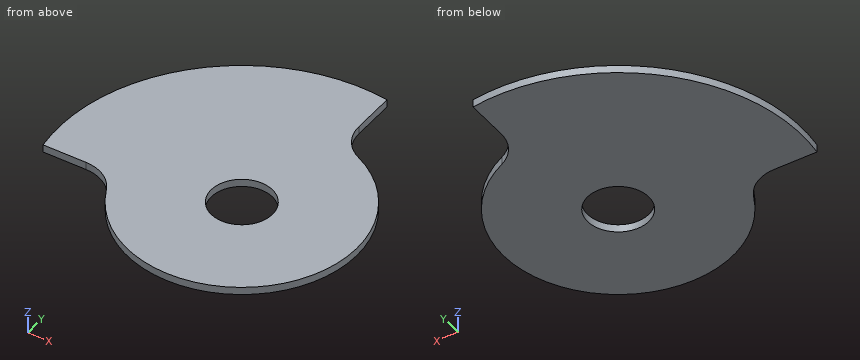
from build123d import *

# Parameters (mm, degrees)
SKETCH_1_R          = 24
EXTRUDE_1_DEPTH     = 1
CUT_EXTRUDE_START   = -1
SKETCH_2_R          = 4
CUT_EXTRUDE_1_DEPTH = 1
FILLET_1_R          = 5
FILLET_2_R          = 5


with BuildPart() as part:
    # 草图1 → 拉伸1 (new body)
    with BuildSketch(Plane.XY):
        Circle(SKETCH_1_R)
    extrude(amount=EXTRUDE_1_DEPTH)

    # 草图2 → 切除-拉伸1 (cut)
    with BuildSketch(Plane.XY.offset(1).offset(CUT_EXTRUDE_START)):
        Circle(SKETCH_2_R)
        with BuildLine():
            Line((-23.743420141, -3.5), (-14.585952146, -3.5))
            ThreePointArc((-14.585952146, -3.5), (10.606601718, -10.606601718), (3.5, 14.585952146))
            Line((3.5, 14.585952146), (3.5, 23.743420141))
            ThreePointArc((3.5, 23.743420141), (16.970562748, -16.970562748), (-23.743420141, -3.5))
        make_face()
    extrude(amount=CUT_EXTRUDE_1_DEPTH, mode=Mode.SUBTRACT)

    # 圆角1
    fillet_1_edges = [part.edges().sort_by_distance(p)[0] for p in [
        (-14.585952146, -3.5, 0.5),
    ]]
    fillet(fillet_1_edges, radius=FILLET_1_R)

    # 圆角2
    fillet_2_edges = [part.edges().sort_by_distance(p)[0] for p in [
        (3.5, 14.585952146, 0.5),
    ]]
    fillet(fillet_2_edges, radius=FILLET_2_R)


solid = part.part
The listing builds one solid part. Answer for the finished solid, in the listing's coordinates (mm). Round coordinates to 2 decimals unless told otherwise and drop trailing zeros. Loops run counter-clockwise (first coordinate to the right, second up) from the corner with the lowest first, then second, coordinate; pieces in that order, holes last. Notation, with made-up numbers: M 33,40.5 L 68,40.5 A20 ccw 68,75.5 Z; hole C 85.5,14.25 d8. An arc over 180 degrees is marked long. Return JSON: item names as keys, results as strings.
Q1. Find section D-D, the plane x = 9. Determine the outline of the cut face in (y, z).
Results list:
{"outline": "M -12,0 L 12,0 L 12,1 L -12,1 Z"}
Q2. Find section C-C, the plane z = 0.5. Determine the outline of the cut face in (x, y) (3 decimals), plus the area to 4 significant figures.
Results list:
{"outline": "M -23.743,-3.5 L -18.104,-3.5 A5 cw -13.578,-6.375 A15 ccw long 6.375,13.578 A5 cw 3.5,18.104 L 3.5,23.743 A24 ccw Z; hole C 0,0 d8", "area": "1,000 mm2"}
Q3. Find section B-B, the plane x = 0. Determine the outline of the cut face in (y, z), plus the area to 3 significant figures.
Results list:
{"outline": "M -15,0 L -4,0 L -4,1 L -15,1 Z; M 4,0 L 24,0 L 24,1 L 4,1 Z", "area": "31.0 mm2"}
Q4. Find the intervals of material crossed by line 1 along Y through (x, z) = (0, 0.5); line 2 along X through (y, z) = (11.5, 0.1); line 3 along Y through (x, z) = (8.5, 0.15), in increasing order. Write a range as from..to.
Results list:
{"line 1": "y = -15..-4, 4..24", "line 2": "x = -21.07..9.63", "line 3": "y = -12.36..12.36"}
Q5. Find section A-A, the plane y = 0. Determine the outline of the cut face in (x, z).
Results list:
{"outline": "M -24,0 L -4,0 L -4,1 L -24,1 Z; M 4,0 L 15,0 L 15,1 L 4,1 Z"}
